Could you check a few things on this model? Use its own coordinates, in mm. Give positions to 0.01 mm unless a question says otherwise; leave off trailing zeros. Loops run counter-clockwise (first coordinate to the right, second up) from the corner with the lowest first, then second, coordinate; pieces in that order, holes last. Notation, with made-up numbers: (-21.5, -11.5) -> (11.5, -11.5) arc R34 ccw to (11.5, 26.5) -> close; hole circle Ø2 at (-14.75, 26.5). An arc over 180 degrees is marked (long way). Write item = value, one per line. Start each with the question number.
1) I need wall thicknesses on probe 1 along X at (y, z) = (2.5, 1.6); probe 2 along X at (y, z) = (3, 4.1); probe 3 along Y at (x, z) = (-250, 2.15). Which ranges of each line are inside material? Lowest first, please. Write a range as from..to.
2) I want a section at A-A (x = -210.5). List the corners of the cut face in (y, z) for me, and give its area (3 significant figures).
3) I'm going to push a flat-ended pin straight in: pin 1 Ø1 at (y, z) = (3.5, 1.5) entering from +X. Where does the tip first touch, or does it pass through?
from build123d import *

# Parameters (mm, degrees)
SKETCH1_W           = 265
SKETCH1_H           = 5
BOSS_EXTRUDE1_DEPTH = 5
SKETCH2_R           = 1
CUT_EXTRUDE1_DEPTH  = 266.094322836
FILLET1_R           = 2


with BuildPart() as part:
    # Sketch1 → Boss-Extrude1 (new body)
    with BuildSketch(Plane.XY):
        with Locations((-132.5, 2.5)):
            Rectangle(SKETCH1_W, SKETCH1_H)
    extrude(amount=BOSS_EXTRUDE1_DEPTH)

    # Sketch2 → Cut-Extrude1 (cut, through all)
    with BuildSketch(Plane.XY.offset(5)):
        with Locations((-250, 2.5)):
            Circle(SKETCH2_R)
        with Locations(Location((-15, 2.5, 0), (0, 0, 180))):
            Circle(SKETCH2_R)
    extrude(amount=-CUT_EXTRUDE1_DEPTH, mode=Mode.SUBTRACT)

    # Fillet1
    # the kernel refuses this fillet: 2 mm, written as the material it takes off along each edge
    with BuildSketch(Plane(origin=(5, 0, 5), x_dir=(0, 0, -1), z_dir=(-1, 0, 0))) as fillet1_piece_1:
        with BuildLine():
            CenterArc((FILLET1_R, -FILLET1_R), FILLET1_R, 90, 90)
            Line((0, -FILLET1_R), (0, 0))
            Line((0, 0), (FILLET1_R, 0))
        make_face()
    extrude(amount=275, mode=Mode.SUBTRACT)
    with BuildSketch(Plane(origin=(-270, 5, 5), x_dir=(0, -1, 0), z_dir=(1, 0, 0))) as fillet1_piece_2:
        with BuildLine():
            CenterArc((FILLET1_R, FILLET1_R), FILLET1_R, 180, 90)
            Line((0, FILLET1_R), (0, 0))
            Line((0, 0), (FILLET1_R, 0))
        make_face()
    extrude(amount=275, mode=Mode.SUBTRACT)


solid = part.part
Answer list:
q1.probe_1 = -265..-251, -249..-16, -14..0
q1.probe_2 = -265..-250.87, -249.13..-15.87, -14.13..0
q1.probe_3 = 0..1.5, 3.5..5
q2.outline = (0, 0) -> (5, 0) -> (5, 3) arc R2 ccw to (3, 5) -> (2, 5) arc R2 ccw to (0, 3) -> close
q2.area = 23.3 mm^2
q3.pin_1 = 0
